```python
from build123d import *

# Parameters (mm, degrees)
F1_DEPTH = 19.05


with BuildPart() as f1:
    # F0 (on Front) → F1 (new body)
    with BuildSketch(Plane.XZ):
        Polygon((3.666174, 6.35), (-3.666174, 6.35), (-7.332348, 0), (-3.666174, -6.35), (3.666174, -6.35), (7.332348, 0), align=None)
        with BuildLine():
            ThreePointArc((1, 3.872983), (0, -4), (-1, 3.872983))
            Line((-1, 3.872983), (-1, 4.872983))
            Line((-1, 4.872983), (1, 4.872983))
            Line((1, 4.872983), (1, 3.872983))
        make_face(mode=Mode.SUBTRACT)
    extrude(amount=F1_DEPTH)


solid = f1.part
```
The model under review builds one solid part; all positions refer to its coordinate system, in mm. A direction names the side the tool comes from. Give positions to 0.01 mm unless a question says otherwise; leave off trailing zeros. Order: outer loops, then holes, each group sorted by start corner. A loop starts at its lowest first (then second) coordinate and runs counter-clockwise, first axis right, second up. Notation, with made-up numbers: (8.5, 52) - (30.5, 52) arc R14 ccw to (30.5, 64) - close; hole circle Ø7 at (-14, 18). An arc over 180 degrees is marked (long way). Use CSV: the item, a comma, the result in double quotes. Start each with the question number.
Q1. We need section D-D, the plane x = -5. Write out the cut boundary in (y, z).
Q2. Tool access review of faces 1 (the flat face through (0, -9, 4.873)), 2 (the flat face through (0, -9, -6.35)): name each direction out of +Z, -Z, +X, -X, +Y, -Y from which nothing blocks a thin tool from reaching the whole face with its end or side.
Q3. We need section A-A, the plane x = 0. Write out the cut boundary in (y, z).
Q4. We need section C-C, the plane z = -0.5. Write out the cut boundary in (x, y), and give its area (3 significant figures).
Q5. To check wall thickness, follow line 1 along Z through (x, y) = (0, -8.25); line 2 along X through (y, z) = (-1.5, 1.75); line 3 along X through (y, z) = (-12.5, -0.5). State the ranges of each line that lie inside material, in increasing order. Write a range as [from, to].
Q6. The part is to be moulded in two halves that separate along X. For faces 3 (the flat face through (3, -19.05, -3)), 4 (the flat face through (1, -9.4, 4.4)), 5 (the flat face through (5.525, -9.392, 3.131)), 6 (the flat face through (-5.525, -9.392, -3.131)), say which applies: +X half, -X half, draft (parallel to the pull), parting line (faces both ways), or undercut.
Q7. We need section B-B, the plane y = -14.5. Write out the cut boundary in (x, z), and give its area (3 significant figures).
Q8. Clearance check with flat-ended pins moving along their axes: pin 1 Ø0.8 at (y, z) = (-9, 4.5) entering from -X; pin 2 Ø1.1 at (y, z) = (-5, 4.5) entering from +X; pin 3 Ø1 at (y, z) = (-11.5, -3.5) entering from -X. State where each tip first meets the part, or that it passes through.
Outcome:
1,outline,"(-19.05, -4.04) - (0, -4.04) - (0, 4.04) - (-19.05, 4.04) - close"
2,face 1,"+Y, -Y"
2,face 2,"-Z, +X, -X, +Y, -Y"
3,outline,"(-19.05, -6.35) - (0, -6.35) - (0, -4) - (-19.05, -4) - close; (-19.05, 4.87) - (0, 4.87) - (0, 6.35) - (-19.05, 6.35) - close"
4,outline,"(-7.04, -19.05) - (-3.97, -19.05) - (-3.97, 0) - (-7.04, 0) - close; (3.97, -19.05) - (7.04, -19.05) - (7.04, 0) - (3.97, 0) - close"
4,area,"117 mm^2"
5,line 1,"z = [-6.35, -4], [4.87, 6.35]"
5,line 2,"x = [-6.32, -3.6], [3.6, 6.32]"
5,line 3,"x = [-7.04, -3.97], [3.97, 7.04]"
6,face 3,"draft"
6,face 4,"undercut"
6,face 5,"+X half"
6,face 6,"-X half"
7,outline,"(-7.33, 0) - (-3.67, -6.35) - (3.67, -6.35) - (7.33, 0) - (3.67, 6.35) - (-3.67, 6.35) - close; hole (-1, 3.87) arc R4 ccw (long way) to (1, 3.87) - (1, 4.87) - (-1, 4.87) - close"
7,area,"87.6 mm^2"
8,pin 1,"stops at x = -4.97"
8,pin 2,"stops at x = 5.05"
8,pin 3,"stops at x = -5.6"
